Geometry check sheet. Reference: the model listing, model coordinates, mm. Give positions to 0.01 mm unless a question says otherwise; leave off trailing zeros. Order: outer loops, then holes, each group sorted by start corner. A loop starts at its lowest first (then second) coordinate and runs counter-clockwise, first axis right, second up. Notation, with made-up numbers: M 50.25,78.25 L 73.25,78.25 A14 ccw 73.25,105.25 Z; hole C 21.5,59.25 d10. An arc over 180 degrees is marked long. Answer as CSV lines item,"result". Start each with the question number.
Q1. Go/stop test with flat-tipped pins: pin 1 (5 mm diameter, centred on x = -77.75, z = -164.25, fed in from +Y); pin 2 (1 mm diameter, centred on x = -30, y = 0.5, fed in from -Z). Record where each tip stops, or that it passes through.
Q2. Section check C-C, the plane x = -114. Record the boundary of the cut face in (y, z), then the cut area to 3 significant figures.
Q3. Thickness scan on line 1 (Z direction, x = -98.25, y = 0.75); line 2 (X direction, y = 0.85, z = -108.25); line 3 (X direction, y = 2.85, z = -124). Record the ranges inside material, lowest first.
Q4. Section check A-A, the plane z = -125. Record the boundary of the cut face in (x, y), then the cut area to 3 significant figures.
Q5. Section check B-B, the plane y = 0.45. Count the separate pieces of the cut face and the enclosed holes in it, then the cut area to 3 significant figures.
```python
from build123d import *

# Parameters (mm, degrees)
SKETCH1_R           = 1.5
BOSS_EXTRUDE1_DEPTH = 3


with BuildPart() as part:
    # Sketch1 → Boss-Extrude1 (new body)
    with BuildSketch(Plane(origin=(0, 0, 0), x_dir=(1, 0, 0), z_dir=(0, 1, 0))):
        with BuildLine():
            Line((-4, 0), (-136, 0))
            ThreePointArc((-136, 0), (-138.828427125, 1.171572875), (-140, 4))
            Line((-140, 4), (-140, 166.25343074))
            ThreePointArc((-140, 166.25343074), (-138.828427125, 169.081857865), (-136, 170.25343074))
            Line((-136, 170.25343074), (-117.588107797, 170.25343074))
            Line((-117.588107797, 170.25343074), (-117.588107797, 114.261134971))
            Line((-117.588107797, 114.261134971), (-92.588107797, 114.261134971))
            Line((-92.588107797, 114.261134971), (-92.588107797, 170.25343074))
            Line((-92.588107797, 170.25343074), (-49.754336385, 170.25343074))
            Line((-49.754336385, 170.25343074), (-49.754336385, 115.66527195))
            Line((-49.754336385, 115.66527195), (-20.860369091, 115.66527195))
            Line((-20.860369091, 115.66527195), (-20.860369091, 170.25343074))
            Line((-20.860369091, 170.25343074), (-4, 170.25343074))
            ThreePointArc((-4, 170.25343074), (-1.171572875, 169.081857865), (0, 166.25343074))
            Line((0, 166.25343074), (0, 4))
            ThreePointArc((0, 4), (-1.171572875, 1.171572875), (-4, 0))
        make_face()
        with Locations((-136, 166.25343074)):
            Circle(SKETCH1_R, mode=Mode.SUBTRACT)
        with Locations((-4, 166.25343074)):
            Circle(SKETCH1_R, mode=Mode.SUBTRACT)
        with Locations((-136, 4)):
            Circle(SKETCH1_R, mode=Mode.SUBTRACT)
        with Locations((-4, 4)):
            Circle(SKETCH1_R, mode=Mode.SUBTRACT)
        with Locations((-8.360369091, 141.5902664)):
            Circle(SKETCH1_R, mode=Mode.SUBTRACT)
        with Locations((-8.360369091, 131.5902664)):
            Circle(SKETCH1_R, mode=Mode.SUBTRACT)
        with Locations((-123.265486726, 62.577470458)):
            Circle(SKETCH1_R, mode=Mode.SUBTRACT)
        with Locations((-123.265486726, 9.24694437)):
            Circle(SKETCH1_R, mode=Mode.SUBTRACT)
        with Locations((-61.946271424, 164.25343074)):
            Circle(SKETCH1_R, mode=Mode.SUBTRACT)
        with Locations((-77.75445726, 164.25343074)):
            Circle(SKETCH1_R, mode=Mode.SUBTRACT)
        with Locations((-131.022006432, 155.660698945)):
            Circle(SKETCH1_R, mode=Mode.SUBTRACT)
        with Locations((-131.022006432, 97.992651369)):
            Circle(SKETCH1_R, mode=Mode.SUBTRACT)
        with Locations((-27.5, 81.5)):
            Circle(SKETCH1_R, mode=Mode.SUBTRACT)
        with Locations((-76.5, 81.5)):
            Circle(SKETCH1_R, mode=Mode.SUBTRACT)
        with Locations((-27.5, 23.5)):
            Circle(SKETCH1_R, mode=Mode.SUBTRACT)
        with Locations((-76.5, 23.5)):
            Circle(SKETCH1_R, mode=Mode.SUBTRACT)
        with Locations((-98.25, 108.25)):
            Circle(SKETCH1_R, mode=Mode.SUBTRACT)
        with Locations((-12.919798313, 108.25)):
            Circle(SKETCH1_R, mode=Mode.SUBTRACT)
        with Locations((-98.25, 1.75)):
            Circle(SKETCH1_R, mode=Mode.SUBTRACT)
        with Locations((-13.615959215, 1.75)):
            Circle(SKETCH1_R, mode=Mode.SUBTRACT)
        with BuildLine():
            Line((-78.053728576, 91.841911577), (-61.946271424, 91.841911577))
            ThreePointArc((-61.946271424, 91.841911577), (-61.196519269, 91.092159423), (-61.946271424, 90.342407268))
            Line((-61.946271424, 90.342407268), (-78.053728576, 90.342407268))
            ThreePointArc((-78.053728576, 90.342407268), (-78.803480731, 91.092159423), (-78.053728576, 91.841911577))
        make_face(mode=Mode.SUBTRACT)
    extrude(amount=BOSS_EXTRUDE1_DEPTH)


solid = part.part
```
Answer block:
1,pin 1,"stops at y = 3"
1,pin 2,"stops at z = -115.67"
2,outline,"M 0,-114.26 L 3,-114.26 L 3,0 L 0,0 Z"
2,area,"343 mm2"
3,line 1,"z = -114.26 to -109.75, -106.75 to -3.25, -0.25 to 0"
3,line 2,"x = -140 to -99.75, -96.75 to -14.42, -11.42 to 0"
3,line 3,"x = -140 to -117.59, -92.59 to -49.75, -20.86 to 0"
4,outline,"M -140,0 L -117.59,0 L -117.59,3 L -140,3 Z; M -92.59,0 L -49.75,0 L -49.75,3 L -92.59,3 Z; M -20.86,0 L 0,0 L 0,3 L -20.86,3 Z"
4,area,"258 mm2"
5,separate pieces,"1"
5,enclosed holes,"21"
5,area,"20,700 mm2"
